Autodesk Inventor part; units mm, degrees
ref_plane "Work Plane6" through (0, 25.4, -165.1) normal (0, 0, 1) x (1, 0, 0)
ref_plane "Work Plane12" through (0, 25.4, 0) normal (0, -1, 0) x (1, 0, 0)
ref_plane "Work Plane14" through (-0.824, -18.8821, -44.9646) normal (1, 0, 0) x (0, 1, 0)
sketch "Sketch1" plane through (0, 0, 0) normal (0, 1, 0) x (-1, 0, 0)
  circle A0 centre (0, 0) radius 152.4
  circle A1 centre (0, 0) radius 165.1
  dimension "d0" = 304.8
  dimension "d1" = 330.2
extrude "Extrusion1" add sketch "Sketch1" along normal blind 152.4
sketch "Sketch2" plane through (0, 0, 0) normal (1, 0, 0) x (0, 1, 0)
  circle A0 centre (100.6077, 0) radius 25.4
  point P0 (0, 0)
  dimension "d4" = 50.8
extrude "Extrusion2" add sketch "Sketch2" along normal mid plane 889
sketch "Sketch4" plane through (0, 152.4, 0) normal (0, 1, 0) x (1, 0, 0)
  circle A0 centre (0, 0) radius 152.4
extrude "Extrusion4" cut sketch "Sketch4" against normal through all
sketch "Sketch5" plane through (0, 152.4, 0) normal (0, 1, 0) x (1, 0, 0)
  circle A0 centre (0, 0) radius 165.1
extrude "Extrusion5" add sketch "Sketch5" along normal blind 50.8 draft -50
ref_plane "Work Plane2" through (75.376, -18.8821, -44.9646) normal (1, 0, 0) x (0, 1, 0)
ref_plane "Work Plane5" through (0, 25.4, 165.1) normal (0, 0, 1) x (1, 0, 0)
sketch "Sketch11" plane through (0, 25.4, 165.1) normal (0, 0, 1) x (1, 0, 0)
  circle A0 centre (0, 75.2094) radius 25.4
  line L0 (165.1, -25.4) -> (-165.1, -25.4)
  point P0 (0, -25.4)
  dimension "d31" = 50.8
  dimension "d32" = 100.6094
extrude "Extrusion11" add sketch "Sketch11" along normal blind 280.543
ref_plane "Work Plane6" through (0, 25.4, -165.1) normal (0, 0, 1) x (1, 0, 0)
sketch "Sketch12" plane through (0, 25.4, -165.1) normal (0, 0, 1) x (1, 0, 0)
  circle A0 centre (0, 75.2094) radius 25.4
  line L0 (165.1, -25.4) -> (-165.1, -25.4)
  point P0 (0, -25.4)
  dimension "d36" = 50.8
  dimension "d37" = 100.6094
extrude "Extrusion12" add sketch "Sketch12" against normal blind 280.543
ref_plane "Work Plane10" through (0, 152.4, 0) normal (0, -1, 0) x (1, 0, 0)
ref_plane "Work Plane9" through (0, 63.5, 0) normal (0, -1, 0) x (1, 0, 0)
sketch "Sketch13" plane through (0, 152.4, 0) normal (0, -1, 0) x (1, 0, 0)
  line L0 (-199.2875, -201.2037) -> (234.7376, -201.2037)
  line L1 (234.7376, -201.2037) -> (234.7376, 210.7848)
  line L2 (234.7376, 210.7848) -> (-199.2875, 210.7848)
  line L3 (-199.2875, 210.7848) -> (-199.2875, -201.2037)
  point P0 (0, 0)
extrude "Extrusion13" cut sketch "Sketch13" against normal blind 127
ref_plane "Work Plane11" through (0, 63.5, 0) normal (0, -1, 0) x (1, 0, 0)
sketch "Sketch15" plane through (0, 63.5, 0) normal (0, -1, 0) x (1, 0, 0)
  line L0 (-509.2014, 528.9036) -> (494.7202, 528.9036)
  line L1 (494.7202, 528.9036) -> (494.7202, -498.4488)
  line L2 (494.7202, -498.4488) -> (-509.2014, -498.4488)
  line L3 (-509.2014, -498.4488) -> (-509.2014, 528.9036)
  point P0 (0, 0)
extrude "Extrusion15" cut sketch "Sketch15" against normal blind 254
ref_plane "Work Plane12" through (0, 25.4, 0) normal (0, -1, 0) x (1, 0, 0)
sketch "Sketch16" plane through (0, 25.4, 0) normal (0, -1, 0) x (1, 0, 0)
  line L0 (-189.4244, 211.7722) -> (231.9916, 211.7722)
  line L1 (231.9916, 211.7722) -> (231.9916, -229.8633)
  line L2 (231.9916, -229.8633) -> (-189.4244, -229.8633)
  line L3 (-189.4244, -229.8633) -> (-189.4244, 211.7722)
  point P0 (0, 0)
extrude "Extrusion16" cut sketch "Sketch16" against normal blind 254
ref_plane "Work Plane14" through (-0.824, -18.8821, -44.9646) normal (1, 0, 0) x (0, 1, 0)
ref_plane "Work Plane13" through (164.276, -18.8821, -44.9646) normal (1, 0, 0) x (0, 1, 0)
ref_plane "Work Plane15" through (0, 25.4, 0) normal (0, -1, 0) x (1, 0, 0)
sketch "Sketch17" plane through (0, 25.4, 0) normal (0, -1, 0) x (1, 0, 0)
  line L0 (-206.305, -203.3787) -> (218.0102, -203.3787)
  line L1 (218.0102, -203.3787) -> (218.0102, 226.7892)
  line L2 (218.0102, 226.7892) -> (-206.305, 226.7892)
  line L3 (-206.305, 226.7892) -> (-206.305, -203.3787)
  point P0 (0, 0)
extrude "Extrusion17" cut sketch "Sketch17" along normal blind 19.05
ref_plane "Work Plane8" through (0, 0, 0) normal (0, -1, 0) x (1, 0, 0)
properties part number "UpperSailCapBottom-ver1-1111-2021"
CAD build for the part. Positions are in the model's coordinates, mm. Round coordinates to 2 decimals unless told otherwise and drop trailing zeros. Loops run counter-clockwise (first coordinate to the right, second up) from the corner with the lowest first, then second, coordinate; pieces in that order, holes last. Notation, with made-up numbers: M -37.75,70.25 L -3.75,70.25 A17 ccw -3.75,92.25 Z; hole C 64.5,83 d11. An arc over 180 degrees is marked long. Use a Markdown table: item, result. Add a question column.
(1) Drill centre lines: line 1 (X direction, y = 4, z = 0); line 2 (Z direction, x = -48.5, y = 1.5). Where is each one in solid material? Low to high.
(2) Pull direction X, two halves, no side cores. Call faces 1 (the face through (35.79, 3.131, 161.174)), 2 (the face through (120.94, 3.13, 92.73)), 3 (the face through (-48, 0, -146)): +X half, -X half, draft (parallel to the pull), parting line (faces both ways), or undercut.
(3) Cut at C-C (y = 4.25). Give the cut face in (x, z), and give its area (3 significant figures).
(4) Cut at B-B (z = 0). Give the cut face in (x, y), and give its area (3 significant figures).
(5) Cut at A-A (x = 0). Give the cut face in (y, z).
(6) Flat gauge pins, fed straight in: pin 1 (2 mm diameter, centred on x = 66, y = 1, fed in from -Z); pin 2 (1 mm diameter, centred on y = 4, z = 115, fed in from +X). Where does each tip first touch, or does it go through?
Geometry says:
| question | item | result |
|---|---|---|
| 1 | line 1 | x = -165.1 to -152.4, 152.4 to 165.1 |
| 1 | line 2 | z = -157.82 to -144.48, 144.48 to 157.82 |
| 2 | face 1 | parting line |
| 2 | face 2 | undercut |
| 2 | face 3 | draft |
| 3 | outline | C 0,0 d330.2; hole C 0,0 d304.8 |
| 3 | area | 12,700 mm² |
| 4 | outline | M -165.1,0 L -152.4,0 L -152.4,6.35 L -165.1,6.35 Z; M 152.4,0 L 165.1,0 L 165.1,6.35 L 152.4,6.35 Z |
| 4 | area | 161 mm² |
| 5 | outline | M 0,-165.1 L 6.35,-165.1 L 6.35,-152.4 L 0,-152.4 Z; M 0,152.4 L 6.35,152.4 L 6.35,165.1 L 0,165.1 Z |
| 6 | pin 1 | stops at z = -151.77 |
| 6 | pin 2 | stops at x = 118.94 |
